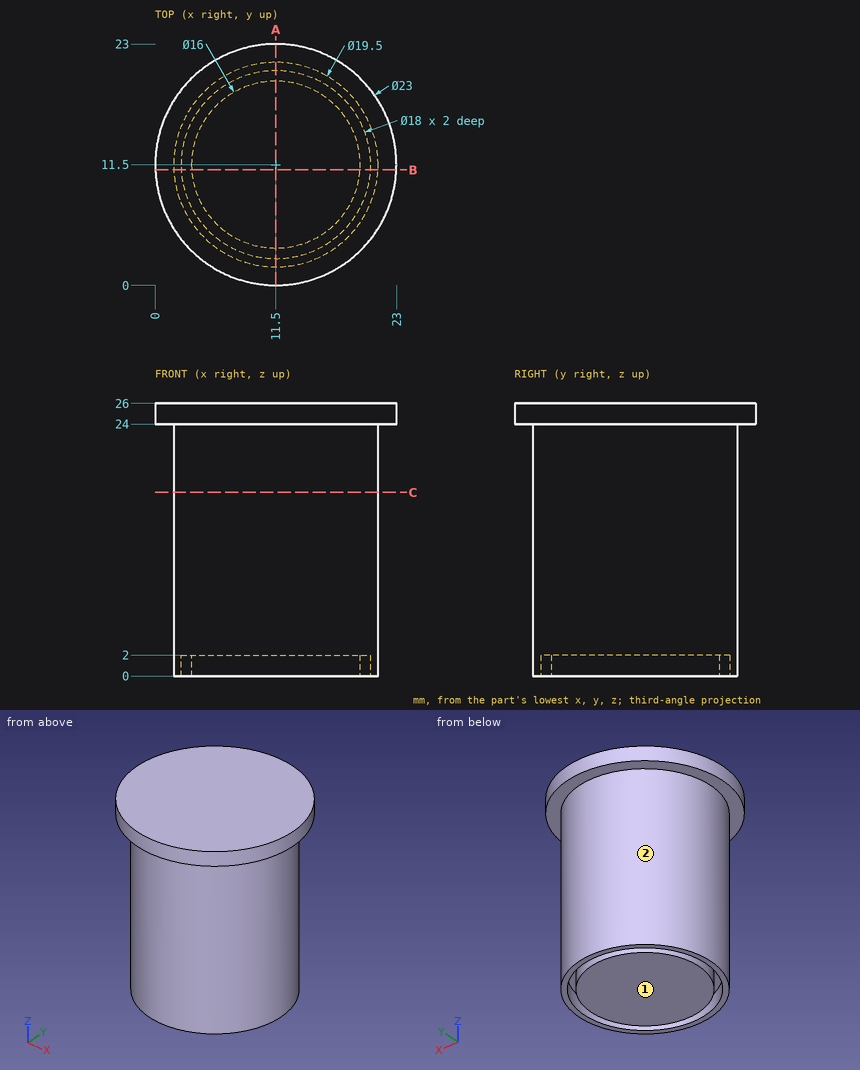
Could you check a few things on this drawing? It's one solid part, dimensions in mm from its lowest x, y, z. A direction names the side the tool comes from. Coordinates: 2 decimals unless noted, no trailing zeros. Write each loop counter-clockwise with the first axis right and the second up, starting at its lowest first coordinate (ties: lowest second). Pieces come first, ordered by that corner, then holes. Notation, with made-up numbers: (74.25, -6.5) - (122.25, -6.5) arc R4 ccw to (122.25, -1.5) - close; hole circle Ø6 at (-30, 24.5). An arc over 180 degrees is marked (long way). Write item = value, one per line.
1) Suppose I cut it at B-B on y = 11. Please give me the cut outline in (x, z).
Result set:
outline = (0.01, 24) - (1.76, 24) - (1.76, 0) - (2.51, 0) - (2.51, 2) - (3.52, 2) - (3.52, 0) - (19.48, 0) - (19.48, 2) - (20.49, 2) - (20.49, 0) - (21.24, 0) - (21.24, 24) - (22.99, 24) - (22.99, 26) - (0.01, 26) - close
2) Will these pins go through, and if not, where does the flat tip stop? pin 1 Ø1.5 at (y, z) = (8.5, 6.5) entering from +X; pin 2 Ø1 at (x, z) = (14.5, 14) entering from +Y; pin 3 Ø1.5 at (x, z) = (5, 14.5) entering from +Y.
Result set:
pin_1 = 20.99
pin_2 = 20.92
pin_3 = 19.37
3) Suppose I cut it at A-A on x = 11.5. Please give me the cut outline in (y, z).
Result set:
outline = (0, 24) - (1.75, 24) - (1.75, 0) - (2.5, 0) - (2.5, 2) - (3.5, 2) - (3.5, 0) - (19.5, 0) - (19.5, 2) - (20.5, 2) - (20.5, 0) - (21.25, 0) - (21.25, 24) - (23, 24) - (23, 26) - (0, 26) - close
4) For the marked faces 1 and 2, which set-ups out of +Z, -Z, +X, -X, +Y, -Y let a thin tool reach every point of the face, with its end or its side?
Result set:
face_1 = -Z, +X, -X, +Y, -Y
face_2 = -Z
5) Please list where these lines run through material, in increasing order: line 1 (Y direction, x = 11.5, z = 1.4); line 2 (Z direction, x = 21, y = 17.5); line 3 (Z direction, x = 9, y = 19.75). Write a range as [from, to].
Result set:
line_1 = [1.75, 2.5], [3.5, 19.5], [20.5, 21.25]
line_2 = [24, 26]
line_3 = [2, 26]
6) Suppose I cut it at C-C on z = 17.5. Please give me the cut outline in (x, y).
Result set:
outline = circle Ø19.5 at (11.5, 11.5)
